Source: CAD feature listing. Evaluate the final solid. Frame: model axes, mm. Face numbers are marked on the shaded views. A direction names the side the tool comes from. Give positions to 0.01 mm unless a question says otherwise; leave off trailing zeros. Loops run counter-clockwise (first coordinate to the right, second up) from the corner with the lowest first, then second, coordinate; pieces in that order, holes last. Notation, with made-up numbers: (15, 22.25) -> (45, 22.25) arc R22 cw to (45, 60.25) -> close; hole circle Ø3 at (82.5, 64.5). An arc over 180 degrees is marked (long way). Return JSON: item names as keys, results as strings. Group by question number.
(1) Draft query along Z for the marked faces 5, 6 and 7. Return one class per face: released by +Z, released by -Z, zero draft, split by the parting line, or undercut.
(2) Cut plane A-A on x = 0. Return loops of the section in (y, z), then the cut area to 3 significant figures.
(3) Access query for the marked faces 1, 2, 3 and 4. Directions: +Z, -Z, +X, -X, +Y, -Y. A direction counts if a zero-diameter tool reaches every point of the face in a straight line with its end or side. Return the directions, or none.
(4) Ray query, line 1 (Z direction, x = 9.75, y = 10.25); line 2 (Y direction, x = 0, z = 11.25); line 3 (X direction, y = -13, z = 5.25). Return the intervals inside material, ascending. Write a range as from..to.
(5) Cut plane C-C on z = 12.25. Return loops of the section in (x, y).
(6) Pin query (flat end, axial travel): pin 1 (1 mm diameter, centred on x = -10.5, y = 7, fed in from -Z); pin 2 (2 mm diameter, centred on x = 13.5, z = 10.5, fed in from +Y); pin 3 (0.8 mm diameter, centred on x = -13, z = 9.5, fed in from -Y); pin 4 (2 mm diameter, centred on y = -9.5, z = 15.5, fed in from -X). Return the tip coordinate at first contact, or that it passes through.
(7) Cut plane D-D on z = 15.5. Return loops of the section in (x, y), then the cut area to 3 significant figures.
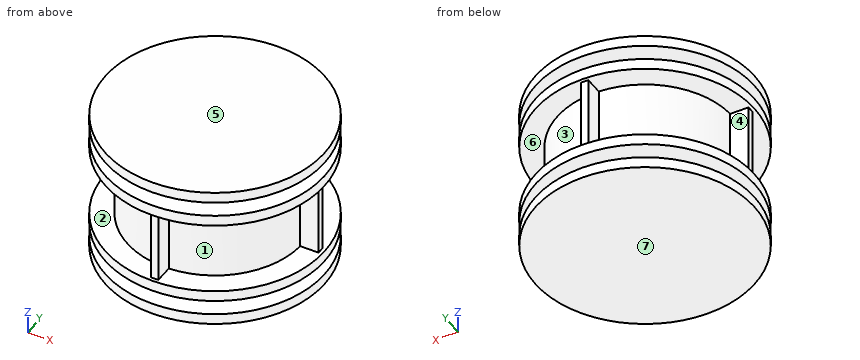
```python
from build123d import *

# Parameters (mm, degrees)
CYLINDER_R               = 12
CYLINDER_DEPTH           = 20
CYLINDER001_R            = 15
CYLINDER001_DEPTH        = 1.5
CYLINDER002_R            = 15
CYLINDER002_DEPTH        = 1.5
CYLINDER003_R            = 15
CYLINDER003_DEPTH        = 1.5
CYLINDER004_R            = 15
CYLINDER004_DEPTH        = 1.5
BOX_W                    = 29
BOX_H                    = 1
BOX_DEPTH                = 10
BOX001_W                 = 29
BOX001_H                 = 1
BOX001_DEPTH             = 10
COMPOUND_PLACEMENT_ANGLE = 90


with BuildPart() as cylinder:
    # Cylinder → Cylinder (new body)
    with BuildSketch(Plane.XY):
        Circle(CYLINDER_R)
    extrude(amount=CYLINDER_DEPTH)


with BuildPart() as cylinder001:
    # Cylinder001 → Cylinder001 (new body)
    with BuildSketch(Plane.XY):
        Circle(CYLINDER001_R)
    extrude(amount=CYLINDER001_DEPTH)


with BuildPart() as cylinder002:
    # Cylinder002 → Cylinder002 (new body)
    with BuildSketch(Plane.XY.offset(3.5)):
        Circle(CYLINDER002_R)
    extrude(amount=CYLINDER002_DEPTH)


with BuildPart() as cylinder003:
    # Cylinder003 → Cylinder003 (new body)
    with BuildSketch(Plane.XY.offset(18.5)):
        Circle(CYLINDER003_R)
    extrude(amount=CYLINDER003_DEPTH)


with BuildPart() as cylinder004:
    # Cylinder004 → Cylinder004 (new body)
    with BuildSketch(Plane.XY.offset(15)):
        Circle(CYLINDER004_R)
    extrude(amount=CYLINDER004_DEPTH)


with BuildPart() as cube:
    # Box → Box (new body)
    with BuildSketch(Plane(origin=(-14.5, -0.5, 5), x_dir=(1, 0, 0), z_dir=(0, 0, 1))):
        with Locations((14.5, 0.5)):
            Rectangle(BOX_W, BOX_H)
    extrude(amount=BOX_DEPTH)


with BuildPart() as basewheel_hollowsides:
    # Box001 → Box001 (new body)
    with BuildSketch(Plane(origin=(-14.5, -0.5, 5), x_dir=(1, 0, 0), z_dir=(0, 0, 1))):
        with Locations((14.5, 0.5)):
            Rectangle(BOX001_W, BOX001_H)
    extrude(amount=BOX001_DEPTH)


with BuildPart() as basewheel_hollowsides_1:
    # Compound placement: moved
    add(basewheel_hollowsides.part.rotate(Axis((0, 0, 0), (0, 0, 1)), COMPOUND_PLACEMENT_ANGLE))

    # Fusion: union Cylinder, Cylinder001, Cylinder002, Cylinder003, Cylinder004, Cube
    add(cylinder.part)
    add(cylinder001.part)
    add(cylinder002.part)
    add(cylinder003.part)
    add(cylinder004.part)
    add(cube.part)


solid = basewheel_hollowsides_1.part
```
Answers:
{
 "1": {"face 5": "released by +Z", "face 6": "undercut", "face 7": "released by -Z"},
 "2": {"outline": "(-15, 0) -> (15, 0) -> (15, 1.5) -> (12, 1.5) -> (12, 3.5) -> (15, 3.5) -> (15, 5) -> (14.5, 5) -> (14.5, 15) -> (15, 15) -> (15, 16.5) -> (12, 16.5) -> (12, 18.5) -> (15, 18.5) -> (15, 20) -> (-15, 20) -> (-15, 18.5) -> (-12, 18.5) -> (-12, 16.5) -> (-15, 16.5) -> (-15, 15) -> (-14.5, 15) -> (-14.5, 5) -> (-15, 5) -> (-15, 3.5) -> (-12, 3.5) -> (-12, 1.5) -> (-15, 1.5) -> close", "area": "566 mm²"},
 "3": {"face 1": "+X, -Y", "face 2": "none", "face 3": "+X, +Y", "face 4": "-X, +Y"},
 "4": {"line 1": "0..1.5, 3.5..5, 15..16.5, 18.5..20", "line 2": "-14.5..14.5", "line 3": "-0.5..0.5"},
 "5": {"outline": "(-14.5, -0.5) -> (-11.99, -0.5) arc R12 ccw to (-0.5, -11.99) -> (-0.5, -14.5) -> (0.5, -14.5) -> (0.5, -11.99) arc R12 ccw to (11.99, -0.5) -> (14.5, -0.5) -> (14.5, 0.5) -> (11.99, 0.5) arc R12 ccw to (0.5, 11.99) -> (0.5, 14.5) -> (-0.5, 14.5) -> (-0.5, 11.99) arc R12 ccw to (-11.99, 0.5) -> (-14.5, 0.5) -> close"},
 "6": {"pin 1": "z = 0", "pin 2": "y = 0.5", "pin 3": "y = -0.5", "pin 4": "x = -12.36"},
 "7": {"outline": "circle Ø30 at (0, 0)", "area": "707 mm²"}
}
